```python
from build123d import *

# Parameters (mm, degrees)
BOSS_EXTRUDE1_DEPTH     = 12.7
SKETCH2_R               = 6.35
SKETCH2_R_2             = 127
SKETCH2_R_3             = 3.81
CUT_EXTRUDE1_DEPTH      = 1
CUT_EXTRUDE1_DEPTH_BACK = 13.7
SKETCH3_W               = 50.8
SKETCH3_H               = 203.2
SKETCH3_W_2             = 203.2
SKETCH3_H_2             = 50.8
CUT_EXTRUDE2_DEPTH      = 1
CUT_EXTRUDE2_DEPTH_BACK = 13.7
FILLET1_R               = 10
FILLET2_R               = 10
SCALE1_SCALE            = 0.5


with BuildPart() as part:
    # Sketch1 → Boss-Extrude1 (new body)
    with BuildSketch(Plane(origin=(0, 0, 0), x_dir=(1, 0, 0), z_dir=(0, 1, 0))):
        Polygon((-203.454, 228.598717139), (203.454, 228.598717139), (228.598717139, 203.454), (228.598717139, -203.454), (203.454, -228.598717139), (-203.454, -228.598717139), (-228.598717139, -203.454), (-228.598717139, 203.454), align=None)
    extrude(amount=BOSS_EXTRUDE1_DEPTH)

    # Sketch2 → Cut-Extrude1 (cut, two sides)
    with BuildSketch(Plane(origin=(0, 12.7, 0), x_dir=(1, 0, 0), z_dir=(0, 1, 0))) as cut_extrude1_sk:
        with Locations((202.555974388, 157.654693783)):
            Circle(SKETCH2_R)
        with Locations((157.654693783, 202.555974388)):
            Circle(SKETCH2_R)
        with Locations((-157.654693783, 202.555974388)):
            Circle(SKETCH2_R)
        with Locations((-202.555974388, 157.654693783)):
            Circle(SKETCH2_R)
        with Locations((-157.654693783, -202.555974388)):
            Circle(SKETCH2_R)
        with Locations((-202.555974388, -157.654693783)):
            Circle(SKETCH2_R)
        with Locations((157.654693783, -202.555974388)):
            Circle(SKETCH2_R)
        with Locations((202.555974388, -157.654693783)):
            Circle(SKETCH2_R)
        Circle(SKETCH2_R_2)
        with Locations((180.105334085, 180.105334085)):
            Circle(SKETCH2_R_3)
        with Locations((122.63169491, 122.63169491)):
            Circle(SKETCH2_R_3)
        with Locations((-180.105334085, 180.105334085)):
            Circle(SKETCH2_R_3)
        with Locations((-122.63169491, 122.63169491)):
            Circle(SKETCH2_R_3)
        with Locations((180.105334085, -180.105334085)):
            Circle(SKETCH2_R_3)
        with Locations((122.63169491, -122.63169491)):
            Circle(SKETCH2_R_3)
        with Locations((-122.63169491, -122.63169491)):
            Circle(SKETCH2_R_3)
        with Locations((-180.105334085, -180.105334085)):
            Circle(SKETCH2_R_3)
    extrude(amount=CUT_EXTRUDE1_DEPTH, mode=Mode.SUBTRACT)
    extrude(cut_extrude1_sk.sketch, amount=-CUT_EXTRUDE1_DEPTH_BACK, mode=Mode.SUBTRACT)

    # Sketch3 → Cut-Extrude2 (cut, two sides)
    with BuildSketch(Plane(origin=(0, 12.7, 0), x_dir=(1, 0, 0), z_dir=(0, 1, 0))) as cut_extrude2_sk:
        with Locations((177.798717139, 0)):
            Rectangle(SKETCH3_W, SKETCH3_H)
        with Locations((0, -177.798717139)):
            Rectangle(SKETCH3_W_2, SKETCH3_H_2)
        with Locations((-177.798717139, 0)):
            Rectangle(SKETCH3_W, SKETCH3_H)
        with Locations((0, 177.798717139)):
            Rectangle(SKETCH3_W_2, SKETCH3_H_2)
    extrude(amount=CUT_EXTRUDE2_DEPTH, mode=Mode.SUBTRACT)
    extrude(cut_extrude2_sk.sketch, amount=-CUT_EXTRUDE2_DEPTH_BACK, mode=Mode.SUBTRACT)

    # Fillet1
    fillet1_edges = [part.edges().sort_by_distance(p)[0] for p in [
        (228.598717139, 6.35, -203.454),
        (228.598717139, 6.35, 203.454),
        (203.454, 6.35, 228.598717139),
        (-203.454, 6.35, 228.598717139),
        (-228.598717139, 6.35, 203.454),
        (-228.598717139, 6.35, -203.454),
        (-203.454, 6.35, -228.598717139),
        (203.454, 6.35, -228.598717139),
    ]]
    fillet(fillet1_edges, radius=FILLET1_R)

    # Fillet2
    fillet2_edges = [part.edges().sort_by_distance(p)[0] for p in [
        (203.198717139, 6.35, -101.6),
        (203.198717139, 6.35, 101.6),
        (152.398717139, 6.35, 101.6),
        (152.398717139, 6.35, -101.6),
        (101.6, 6.35, 203.198717139),
        (-101.6, 6.35, 203.198717139),
        (-101.6, 6.35, 152.398717139),
        (101.6, 6.35, 152.398717139),
        (-203.198717139, 6.35, 101.6),
        (-203.198717139, 6.35, -101.6),
        (-152.398717139, 6.35, -101.6),
        (-152.398717139, 6.35, 101.6),
        (-101.6, 6.35, -203.198717139),
        (101.6, 6.35, -203.198717139),
        (101.6, 6.35, -152.398717139),
        (-101.6, 6.35, -152.398717139),
    ]]
    fillet(fillet2_edges, radius=FILLET2_R)


with BuildPart() as part_1:
    # Scale1: scaled about (0, 6.35, 0)
    add(part.part.scale(SCALE1_SCALE).moved(Location((0, 3.175, 0))))


solid = part_1.part
```
Build history of the part. All positions in model axes, mm. A direction names the side the tool comes from. Coordinates: 2 decimals unless noted, no trailing zeros. Order: outer loops, then holes, each group sorted by start corner. A loop starts at its lowest first (then second) coordinate and runs counter-clockwise, first axis right, second up. Notation, with made-up numbers: M -37.75,41.5 L -27.75,41.5 A33 cw -27.75,80.5 Z; hole C 26,-19 d6. An arc over 180 degrees is marked long. One line per question, with ' | ' between items. Start each with the question number.
1. Mould opens along Z. For faces 3 (the face through (77.7, 6.31, -49.37)), 4 (the face through (-108.081, 6.306, -107.946)), 5 (the face through (-50.8, 6, 89)), 6 (the face through (-107.946, 6.306, 108.081)) say: +Z half, -Z half, draft (parallel to the pull), parting line (faces both ways), or undercut.
2. Cut at C-C (z = -54). Write the cut outline in (x, y) (3 decimals).
3. Cut at D-D (y = 6). Count the separate pieces of the cut face and the enclosed holes in it, plus the area to 3 significant figures.
4. Flat gauge pins, fed straight in: P1, Ø3, axis at x = -90.05, z = 90.05, coming from the -Y side; P2, Ø4.5, axis at x = -90.05, z = -90.05, coming from the -Y side (3 decimals). Where does each tip first touch, or does it go through?
5. Cut at A-A (x = 0). Write the cut outline in (y, z) (3 decimals).
6. Cut at B-B (z = 0). Write the cut outline in (x, y) (3 decimals).
7. Wall check: line 1 along Z through (x, y) = (-22.5, 5.25); line 2 along Z through (x, y) = (-83.5, 7); line 3 along X through (y, z) = (8, -98.5). Give the ranges that are in metal, low to high. Write a range as [from, to].
8. Tool access for faces 1 (the face through (-50.8, 6, -89)), 2 (the face through (108.081, 6.306, 107.946)): list every direction of +Z, -Z, +X, -X, +Y, -Y with a clear straight run to the whole face (end or side of a thin tool).
The answers:
1) face 3: undercut | face 4: -Z half | face 5: undercut | face 6: +Z half
2) outline: M -114.299,3.175 L -33.41,3.175 L -33.41,9.525 L -114.299,9.525 Z; M 33.41,3.175 L 114.299,3.175 L 114.299,9.525 L 33.41,9.525 Z
3) separate pieces: 1 | enclosed holes: 21 | area: 28,700 mm2
4) P1: passes through | P2: stops at y = 3.175
5) outline: M 3.175,-114.299 L 9.525,-114.299 L 9.525,-101.599 L 3.175,-101.599 Z; M 3.175,-76.199 L 9.525,-76.199 L 9.525,-63.5 L 3.175,-63.5 Z; M 3.175,63.5 L 9.525,63.5 L 9.525,76.199 L 3.175,76.199 Z; M 3.175,101.599 L 9.525,101.599 L 9.525,114.299 L 3.175,114.299 Z
6) outline: M -114.299,3.175 L -101.599,3.175 L -101.599,9.525 L -114.299,9.525 Z; M -76.199,3.175 L -63.5,3.175 L -63.5,9.525 L -76.199,9.525 Z; M 63.5,3.175 L 76.199,3.175 L 76.199,9.525 L 63.5,9.525 Z; M 101.599,3.175 L 114.299,3.175 L 114.299,9.525 L 101.599,9.525 Z
7) line 1: z = [-114.3, -101.6], [-76.2, -59.38], [59.38, 76.2], [101.6, 114.3] | line 2: z = [-114.3, -50.8], [50.8, 114.3] | line 3: x = [-114.3, -80.36], [-77.29, -50.42], [50.42, 77.29], [80.36, 114.3]
8) face 1: +Y, -Y | face 2: +Z, +X, +Y, -Y
